```python
from build123d import *


with BuildPart() as part:
    # Varredura1: sweep along a path in Esboço2
    with BuildLine(Plane(origin=(0, 0, 0), x_dir=(1, 0, 0), z_dir=(0, 1, 0))) as varredura1_path:
        Line((0, -750), (0, 750))
        ThreePointArc((0, 750), (72.930411485, 926.069588515), (249, 999))
        Line((249, 999), (549, 999))
        ThreePointArc((549, 999), (725.069588515, 926.069588515), (798, 750))
        Line((798, 750), (798, -750))
        ThreePointArc((798, -750), (725.069588515, -926.069588515), (549, -999))
        Line((549, -999), (249, -999))
        ThreePointArc((249, -999), (72.930411485, -926.069588515), (0, -750))
    # Esboço1 → Varredura1 (sweep)
    with BuildSketch(Plane.XY):
        Polygon((0, 11.228855685), (8.980256121, 2.248599564), (6.731656557, 0), (0, 6.731656557), (-6.731656557, 0), (-8.980256121, 2.248599564), align=None)
    sweep(path=varredura1_path.line)


solid = part.part
```
The listing builds one solid part. Answer for the finished solid, in the listing's coordinates (mm). A direction names the side the tool comes from. Give positions to 0.01 mm unless a question says otherwise; leave off trailing zeros. Loops run counter-clockwise (first coordinate to the right, second up) from the corner with the lowest first, then second, coordinate; pieces in that order, holes last. Notation, with made-up numbers: (62.5, 72) - (114.5, 72) arc R23 ccw to (114.5, 86) - close; hole circle Ø5 at (74.25, -5). An arc over 180 degrees is marked (long way). Return JSON: item names as keys, results as strings. Group by question number.
1. Find section A-A (z = -261.5). Write down the section's boundary in (x, y), then the cut area to 3 significant figures.
2. Straight lines are drawn through the part: line 1 (Z direction, x = 150.5, y = 4.5); line 2 (Z direction, x = 49, y = 2); line 3 (X direction, y = 2.25, z = 810). For each, find the intervals that lie inside material, in ascending order. Write a range as [from, to].
3. Which of the six approach directions +Z, -Z, +X, -X, +Y, -Y give full straight-line access (tool end or side, diameter ignored) to faces 1 (the conical face through (717.2, 2.8, -922)), 2 (the conical face through (81.08, 2.14, 921.65)), 3 (the conical face through (74.484, 10.667, 928.396))?
4. Determine the mould class of faces 4 (the conical face through (731.88, 0.11, 928.91)), 5 (the conical face through (66.12, 0.11, -928.91)), 6 (the conical face through (79.356, 0.327, 923.416)) for opening direction X: pulls with the +X half, pulls with the -X half, needs draft (parallel to the pull), parting line crosses it, or undercut.
5. Given pin 1 Ø6 at (y, z) = (5, 453) entering from -X; pin 2 Ø4 at (x, y) = (519.5, 7.5) entering from -Z; pin 3 Ø4 at (y, z) = (6, -139) entering from +X, each flat-ended and moving along its own axis, determine where each tip first touches the part or whether it passes through.
Verdict:
{
 "1": {"outline": "(-8.98, 2.25) - (-6.73, 0) - (0, 6.73) - (6.73, 0) - (8.98, 2.25) - (0, 11.23) - close; (789.02, 2.25) - (791.27, 0) - (798, 6.73) - (804.73, 0) - (806.98, 2.25) - (798, 11.23) - close", "area": "141 mm^2"},
 "2": {"line 1": "z = [-986, -981.12], [-976.26, -971.34], [971.34, 976.26], [981.12, 986]", "line 2": "z = [-912.56, -906.14], [-890.24, -883.15], [883.15, 890.24], [906.14, 912.56]", "line 3": "x = [-1.9, 2.72], [11.96, 16.6], [781.4, 786.04], [795.28, 799.9]"},
 "3": {"face 1": "+Y", "face 2": "-Y", "face 3": "+Z, -X, +Y"},
 "4": {"face 4": "pulls with the +X half", "face 5": "pulls with the -X half", "face 6": "undercut"},
 "5": {"pin 1": "stops at x = -8.98", "pin 2": "stops at z = -1004.73", "pin 3": "stops at x = 805.23"}
}
